Read the model definition and answer for the solid it produces. Units are mm, in the model's axes. A direction names the side the tool comes from. Coordinates: 2 decimals unless noted, no trailing zeros. Order: outer loops, then holes, each group sorted by start corner. A loop starts at its lowest first (then second) coordinate and runs counter-clockwise, first axis right, second up. Notation, with made-up numbers: (-38.5, 56.5) -> (-28.5, 56.5) arc R9 ccw to (-28.5, 69.5) -> close; hole circle Ø5 at (39.25, 63.25). An arc over 180 degrees is marked (long way). Use CSV: the item, a comma, the result in double quotes.
```python
from build123d import *

# Parameters (mm, degrees)
SKETCH2_R               = 17.78
CUT_EXTRUDE1_DEPTH      = 51.816
CUT_EXTRUDE2_DEPTH      = 68.23495628
CUT_EXTRUDE2_DEPTH_BACK = 68.23495628
SKETCH3_R               = 6.35
CUT_EXTRUDE3_START      = -18.796
SKETCH4_W               = 22.352
SKETCH4_H               = 19.05
CUT_EXTRUDE3_DEPTH      = 49.438956346
CUT_EXTRUDE4_DEPTH      = 68.23495628


with BuildPart() as part:
    # Sketch1 → Revolve1 (revolve)
    with BuildSketch(Plane.XY, mode=Mode.PRIVATE) as revolve1_sk:
        with BuildLine():
            Line((0, 0), (22.225, 0))
            Line((22.225, 0), (22.225, 44.196))
            Line((22.225, 44.196), (19.685, 44.196))
            Line((19.685, 44.196), (19.685, 46.736))
            Line((19.685, 46.736), (22.225, 46.736))
            Line((22.225, 46.736), (22.225, 49.276))
            Line((22.225, 49.276), (19.685, 49.276))
            Line((19.685, 49.276), (19.685, 51.816))
            Line((19.685, 51.816), (22.225, 51.816))
            Line((22.225, 51.816), (22.225, 59.436))
            Line((22.225, 59.436), (12.712693656, 59.436))
            ThreePointArc((12.712693656, 59.436), (6.387986381, 58.484288237), (0, 58.166))
            Line((0, 58.166), (0, 0))
        make_face()
    revolve(revolve1_sk.sketch.rotate(Axis((0, 58.166, 0), (0, -1, 0)), 180), axis=Axis((0, 58.166, 0), (0, -1, 0)))

    # Sketch2 → Cut-Extrude1 (cut)
    with BuildSketch(Plane.XZ):
        Circle(SKETCH2_R)
    extrude(amount=-CUT_EXTRUDE1_DEPTH, mode=Mode.SUBTRACT)

    # Sketch3 → Cut-Extrude2 (cut, two sides: drawn at the far end of the back side and taken through both)
    with BuildSketch(Plane.XY.offset(-CUT_EXTRUDE2_DEPTH_BACK)):
        with Locations((0, 30.48)):
            Circle(SKETCH3_R)
    extrude(amount=CUT_EXTRUDE2_DEPTH + CUT_EXTRUDE2_DEPTH_BACK, mode=Mode.SUBTRACT)

    # Sketch4 → Cut-Extrude3 (cut, through all)
    with BuildSketch(Plane.XY.offset(CUT_EXTRUDE3_START)):
        with Locations((0, 30.48)):
            Rectangle(SKETCH4_W, SKETCH4_H)
    cut_extrude3 = extrude(amount=-CUT_EXTRUDE3_DEPTH, mode=Mode.SUBTRACT)

    # Mirror1: Cut-Extrude3 across plane
    add(cut_extrude3.mirror(Plane.XY), mode=Mode.SUBTRACT)

    # Sketch5 → Cut-Extrude4 (cut, symmetric)
    with BuildSketch(Plane.XY):
        with BuildLine():
            Line((6.223, 0), (8.503897348, 3.420061294))
            ThreePointArc((8.503897348, 3.420061294), (9.876155028, 4.665440061), (11.673642553, 5.116104025))
            Line((11.673642553, 5.116104025), (22.225, 5.116104025))
            Line((22.225, 5.116104025), (22.225, 0))
            Line((22.225, 0), (6.223, 0))
        make_face()
    cut_extrude4 = extrude(amount=CUT_EXTRUDE4_DEPTH, both=True, mode=Mode.SUBTRACT)

    # Mirror2: Cut-Extrude4 across plane
    add(cut_extrude4.mirror(Plane(origin=(0, 0, 0), x_dir=(0, 0, 1), z_dir=(1, 0, 0))), mode=Mode.SUBTRACT)


solid = part.part
```
Item 1: Find section D-D, the plane x = 0. Give the number of separate pieces and of enclosed holes in the cut face, then the cut area to 3 significant figures.
Return value:
separate pieces,"3"
enclosed holes,"0"
area,"596 mm^2"
Item 2: The mould has two halves that part along X. Classify faces 5 (the flat face through (-7.35, 1.69, -18.44)), 6 (the cylindrical face through (16.4, 55.7, -15)), 7 (the cylindrical face through (9.85, 4.65, -16.92)), 8 (the flat face through (0, 40.005, -20)): +X half, -X half, draft (parallel to the pull), parting line (faces both ways), or undercut.
Return value:
face 5,"-X half"
face 6,"parting line"
face 7,"+X half"
face 8,"undercut"
Item 3: Each of these flat-tipped pins is pushed along its axis until it touches: P1, Ø8, axis at y = 41.5, z = -17, coming from the -X side; P2, Ø21.5, axis at x = 0, z = 0, coming from the +Y side; P3, Ø1, axis at y = 47.5, z = 17.5, coming from the +X side. Where does it stop, or does it pass through?
Return value:
P1,"stops at x = -18.03"
P2,"stops at y = 59.07"
P3,"stops at x = 14.32"
Item 4: Find section B-B, the plane z = 0. Give the vertices of the cut face in (x, y) (3 decimals).
Return value:
outline,"(-22.225, 5.116) -> (-17.78, 5.116) -> (-17.78, 51.816) -> (17.78, 51.816) -> (17.78, 5.116) -> (22.225, 5.116) -> (22.225, 44.196) -> (19.685, 44.196) -> (19.685, 46.736) -> (22.225, 46.736) -> (22.225, 49.276) -> (19.685, 49.276) -> (19.685, 51.816) -> (22.225, 51.816) -> (22.225, 59.436) -> (12.713, 59.436) arc R64.262 cw to (-12.713, 59.436) -> (-22.225, 59.436) -> (-22.225, 51.816) -> (-19.685, 51.816) -> (-19.685, 49.276) -> (-22.225, 49.276) -> (-22.225, 46.736) -> (-19.685, 46.736) -> (-19.685, 44.196) -> (-22.225, 44.196) -> close"
Item 5: Straight lines are drawn through the part: line 1 along Z through (x, y) = (0, 11.5) (3 decimals); line 2 along Y through (x, z) = (0, 18); line 3 along Y through (x, z) = (0.5, 15). For each, find the intervals that lie inside material, in ascending order.
Return value:
line 1,"z = -22.225 to -17.78, 17.78 to 22.225"
line 2,"y = 0 to 24.13, 36.83 to 59.44"
line 3,"y = 51.82 to 59.44"
Item 6: A tool of negligible diameter and unlimited length cuts with its end or side. For faces 1 (the flat face through (0, 37, -18.796)), 2 (the flat face through (-2, 51.816, 20)), 3 (the cylindrical face through (-6.344, 30.759, 17.929)), 4 (the flat face through (0, 37, 18.796)), from which of +Z, -Z, +X, -X, +Y, -Y can it reach the whole face along a straight path? Write none if from no direction.
Return value:
face 1,"-Z"
face 2,"none"
face 3,"+Z, -Z"
face 4,"+Z"
Item 7: Find section A-A, the plane y = 30.48. Give the vertices of the cut face in (x, z) (3 decimals).
Return value:
outline,"(-11.176, -19.211) -> (-11.176, -18.796) -> (-6.35, -18.796) -> (-6.35, -16.607) arc R17.78 cw to (-6.35, 16.607) -> (-6.35, 18.796) -> (-11.176, 18.796) -> (-11.176, 19.211) arc R22.225 ccw to start; (6.35, -18.796) -> (11.176, -18.796) -> (11.176, -19.211) arc R22.225 ccw to (11.176, 19.211) -> (11.176, 18.796) -> (6.35, 18.796) -> (6.35, 16.607) arc R17.78 cw to (6.35, -16.607) -> close"
